```python
from build123d import *

# Parameters (mm, degrees)
F0_W      = 80
F0_H      = 30
F1_DEPTH  = 7
F2_R      = 11
F3_DEPTH  = 7.001
F4_SIZE   = 10
F5_R      = 5
F6_R      = 9.5
F7_DEPTH  = 7.001
F8_W      = 2
F8_H      = 30
F9_DEPTH  = 2
F10_W     = 2
F10_H     = 30
F11_DEPTH = 2


with BuildPart() as f1:
    # F0 (on Top) → F1 (new body)
    with BuildSketch(Plane.XY):
        Rectangle(F0_W, F0_H)
    extrude(amount=F1_DEPTH)

    # F2 (on face) → F3 (cut, through all)
    with BuildSketch(Plane.XY.offset(7)):
        Circle(F2_R)
    extrude(amount=-F3_DEPTH, mode=Mode.SUBTRACT)

    # F4
    f4_edges = [f1.edges().sort_by_distance(p)[0] for p in [
        (-40, 15, 3.5),
        (40, -15, 3.5),
        (40, 15, 3.5),
        (-40, -15, 3.5),
    ]]
    chamfer(f4_edges, length=F4_SIZE)

    # F5
    f5_edges = [f1.edges().sort_by_distance(p)[0] for p in [
        (-30, 15, 3.5),
        (-30, -15, 3.5),
        (30, -15, 3.5),
        (30, 15, 3.5),
    ]]
    fillet(f5_edges, radius=F5_R)

    # F6 (on face) → F7 (cut, through all)
    with BuildSketch(Plane.XY.offset(7)):
        with Locations((29.84234935, 0)):
            Circle(F6_R)
        with Locations((-29.84234935, 0)):
            Circle(F6_R)
    extrude(amount=-F7_DEPTH, mode=Mode.SUBTRACT)

    # F8 (on face) → F9 (cut)
    with BuildSketch(Plane.XY.offset(7)):
        with Locations((16.7006367594, 0)):
            Rectangle(F8_W, F8_H)
        with Locations((-16.7006367594, 0)):
            Rectangle(F8_W, F8_H)
    extrude(amount=-F9_DEPTH, mode=Mode.SUBTRACT)

    # F10 (on face) → F11 (cut)
    with BuildSketch(Plane(origin=(0, 0, 0), x_dir=(1, 0, 0), z_dir=(0, 0, -1))):
        with Locations((16.6785700023, 0)):
            Rectangle(F10_W, F10_H)
        with Locations((-16.6785700023, 0)):
            Rectangle(F10_W, F10_H)
    extrude(amount=-F11_DEPTH, mode=Mode.SUBTRACT)


solid = f1.part
```
The model under review builds one solid part; all positions refer to its coordinate system, in mm. A direction names the side the tool comes from. Give positions to 0.01 mm unless a question says otherwise; leave off trailing zeros. Write each loop counter-clockwise with the first axis right and the second up, starting at its lowest first coordinate (ties: lowest second). Pieces come first, ordered by that corner, then holes. Notation, with made-up numbers: (-36.75, 64) - (8.25, 64) arc R22 ccw to (8.25, 73) - close; hole circle Ø9 at (-8.5, -2.75). An arc over 180 degrees is marked (long way). Answer in a Markdown table with one row per item. Add a question column.
1. We need section C-C on z = 3.5. Write out the cut boundary in (x, y), then the cut area to 3 significant figures.
2. We need section A-A on y = 0. State how many separate pieces and enclosed holes the cut face has, then the cut area to 3 significant figures.
3. Wall thickness on line 1 along Y through (x, z) = (0, 1.5); line 2 along X through (y, z) = (8.5, 5.75) (3 decimals); line 3 along X through (y, z) = (-3.75, 4): over which ranges is each line inside the solid? List them lowest first. Write a range as [from, to].
4. Draft analysis for pull direction X (two halves, no side actions). For faces 4 (the cylindrical face through (-29.87, -14.61, 3.55)), 5 (the flat face through (-19, 0, 7)), 6 (the flat face through (17.701, 0, 6)), 7 (the flat face through (-15.701, 0, 6)), state which applies: +X half, -X half, draft (parallel to the pull), parting line (faces both ways), or undercut.
5. We need section B-B on x = 0. Write out the cut boundary in (y, z).
6. Insertion check: P1, Ø1, axis at x = -16.5, y = -6, coming from the -Z side; P2, Ø0.6, axis at x = 16.5, y = -6.5, coming from the +Z side; P3, Ø2, axis at y = 6.5, z = 6.5, coming from the -X side. Each pin has a flat end and moves straight along its axis. Give the tip position at first contact, or say it passes through.
7. Tool access review of faces 1 (the flat face through (-11, -3, 7)), 2 (the flat face through (-17, 0, 2)), 3 (the flat face through (-17, 0, 5)): name each direction out of +Z, -Z, +X, -X, +Y, -Y from which nothing blocks a thin tool from reaching the whole face with its end or side.
8. We need section D-D on x = 34.5. Write out the cut boundary in (y, z).
Ans:
| question | item | result |
|---|---|---|
| 1 | outline | (-40, -5) - (-31.46, -13.54) arc R5 ccw to (-27.93, -15) - (27.93, -15) arc R5 ccw to (31.46, -13.54) - (40, -5) - (40, 5) - (31.46, 13.54) arc R5 ccw to (27.93, 15) - (-27.93, 15) arc R5 ccw to (-31.46, 13.54) - (-40, 5) - close; hole circle Ø19 at (-29.84, 0); hole circle Ø22 at (0, 0); hole circle Ø19 at (29.84, 0) |
| 1 | area | 1,250 mm^2 |
| 2 | separate pieces | 4 |
| 2 | enclosed holes | 0 |
| 2 | area | 124 mm^2 |
| 3 | line 1 | y = [-15, -11], [11, 15] |
| 3 | line 2 | x = [-36.5, -34.085], [-25.6, -17.701], [-15.701, -6.982], [6.982, 15.701], [17.701, 25.6], [34.085, 36.5] |
| 3 | line 3 | x = [-40, -38.57], [-21.11, -10.34], [10.34, 21.11], [38.57, 40] |
| 4 | face 4 | -X half |
| 4 | face 5 | draft |
| 4 | face 6 | undercut |
| 4 | face 7 | undercut |
| 5 | outline | (-15, 0) - (-11, 0) - (-11, 7) - (-15, 7) - close; (11, 0) - (15, 0) - (15, 7) - (11, 7) - close |
| 6 | P1 | stops at z = 2 |
| 6 | P2 | stops at z = 5 |
| 6 | P3 | stops at x = -39.5 |
| 7 | face 1 | +Z, +X, -X, +Y, -Y |
| 7 | face 2 | -Z, +Y, -Y |
| 7 | face 3 | +Z, +Y, -Y |
| 8 | outline | (-10.5, 0) - (-8.28, 0) - (-8.28, 7) - (-10.5, 7) - close; (8.28, 0) - (10.5, 0) - (10.5, 7) - (8.28, 7) - close |
